The model under review builds one solid part; all positions refer to its coordinate system, in mm. A direction names the side the tool comes from. Round coordinates to 2 decimals unless told otherwise and drop trailing zeros. Write each loop counter-clockwise with the first axis right and the second up, starting at its lowest first coordinate (ties: lowest second). Pieces come first, ordered by that corner, then holes. Notation, with made-up numbers: M -25.5,31.5 L -5.5,31.5 A28 cw -5.5,56.5 Z; hole C -11.75,30 d10. An arc over 180 degrees is marked long. Write item = value, one per line. Start each with the question number.
Item 1: For pin 1 Ø4 at (x, z) = (-106, -24.5) entering from -Y (3 decimals); pin 2 Ø14.5 at (x, y) = (-106, -23) entering from -Z (3 decimals), all flat-tipped, find the tip position at first contact; note any pin that passes through.
Item 2: Take a section at A-A, the plane x = -50. Give the boundary of the cut face in (y, z) (3 decimals), plus the area to 3 significant figures.
Item 3: The part is to be moulded in two halves that separate along Z. For faces 1 (the cylindrical face through (-53.485, -11.949, -1.61)), 2 (the flat face through (3, -20, 0)), 3 (the flat face through (3, -21, -3.175)), 4 (the cylindrical face through (2.86, -1.61, -24.96)), say which applies: +Z half, -Z half, draft (parallel to the pull), parting line (faces both ways), or undercut.
Item 4: Take a section at B-B, the plane x = 109. Give the boundary of the cut face in (y, z) (3 decimals).
Item 5: To check wall thickness, follow line 1 along Y through (x, z) = (-182.5, -12) (3 decimals); line 2 along Y through (x, z) = (-204, -1). State the ranges of each line that lie inside material, in increasing order.
Item 6: Tool access review of faces 5 (the cylindrical face through (-52.172, -45.633, -1.61)), 6 (the flat face through (3, -3.175, -27)): name each direction out of +Z, -Z, +X, -X, +Y, -Y from which nothing blocks a thin tool from reaching the whole face with its end or side.
from build123d import *

# Parameters (mm, degrees)
BOSS_EXTRUDE1_DEPTH = 214.63
SKETCH2_R           = 2.5
SKETCH2_R_2         = 3.57
CUT_EXTRUDE1_DEPTH  = 223.403254304
CUT_EXTRUDE2_DEPTH  = 3.175
SKETCH4_R           = 2.5
CUT_EXTRUDE3_DEPTH  = 3.175
CUT_EXTRUDE4_REACH  = 224.131
SKETCH5_R           = 9.525
SKETCH6_R           = 2.6
CUT_EXTRUDE5_DEPTH  = 3.175


with BuildPart() as part:
    # Sketch1 → Boss-Extrude1 (new, symmetric)
    with BuildSketch(Plane(origin=(0, 0, 0), x_dir=(0, 0, -1), z_dir=(1, 0, 0))):
        Polygon((0, 0), (31.75, 0), (31.75, -3.175), (3.175, -3.175), (3.175, -50.8), (0, -50.8), align=None)
    extrude(amount=BOSS_EXTRUDE1_DEPTH, both=True)

    # Sketch2 → Cut-Extrude1 (cut, through all)
    with BuildSketch(Plane(origin=(0, 0, -3.175), x_dir=(-1, 0, 0), z_dir=(0, 0, -1))):
        with Locations(Location((-50, -11.175, 0), (0, 0, 90))):
            Circle(SKETCH2_R)
        with Locations(Location((50, -11.175, 0), (0, 0, 90))):
            Circle(SKETCH2_R_2)
        with Locations(Location((50, -42.8, 0), (0, 0, 90))):
            Circle(SKETCH2_R_2)
        with Locations(Location((-50, -42.8, 0), (0, 0, 90))):
            Circle(SKETCH2_R)
    extrude(amount=-CUT_EXTRUDE1_DEPTH, mode=Mode.SUBTRACT)

    # Sketch3 → Cut-Extrude2 (cut)
    with BuildSketch(Plane(origin=(0, 0, -3.175), x_dir=(-1, 0, 0), z_dir=(0, 0, -1))):
        Polygon((214.63, -50.8), (100.33, -50.8), (214.63, -23.175), align=None)
        Polygon((-214.63, -23.175), (-214.63, -50.8), (-100.33, -50.8), align=None)
    extrude(amount=-CUT_EXTRUDE2_DEPTH, mode=Mode.SUBTRACT)

    # Sketch4 → Cut-Extrude3 (cut)
    with BuildSketch(Plane(origin=(0, 0, 0), x_dir=(1, 0, 0), z_dir=(0, 1, 0))):
        with Locations(Location((-204.63, 11.176, 0), (0, 0, 270))):
            Circle(SKETCH4_R)
        with Locations(Location((-204.63, 25.176, 0), (0, 0, 270))):
            Circle(SKETCH4_R)
        with Locations(Location((204.63, 25.176, 0), (0, 0, 90))):
            Circle(SKETCH4_R)
        with Locations(Location((204.63, 11.176, 0), (0, 0, 90))):
            Circle(SKETCH4_R)
    extrude(amount=-CUT_EXTRUDE3_DEPTH, mode=Mode.SUBTRACT)

    # Sketch5 → Cut-Extrude4 (cut, up to next)
    with BuildSketch(Plane.XZ.offset(3.175), mode=Mode.PRIVATE) as cut_extrude4_sk1:
        with Locations(Location((0, -15.875, 0), (0, 0, 270))):
            Circle(SKETCH5_R)
    cut_extrude4_tool1 = extrude(cut_extrude4_sk1.sketch, amount=-CUT_EXTRUDE4_REACH, mode=Mode.PRIVATE) & part.part
    add(cut_extrude4_tool1.solids().sort_by_distance((0, -3.175, -15.875))[0], mode=Mode.SUBTRACT)

    # Sketch6 → Cut-Extrude5 (cut)
    with BuildSketch(Plane.XY):
        with Locations((204.63, -13.175000066)):
            Circle(SKETCH6_R)
        with Locations(Location((-204.63, -13.175000066, 0), (0, 0, 270))):
            Circle(SKETCH6_R)
    extrude(amount=-CUT_EXTRUDE5_DEPTH, mode=Mode.SUBTRACT)


solid = part.part
Response values:
q1.pin_1 = -3.175
q1.pin_2 = -3.175
q2.outline = M -50.8,-3.175 L -46.37,-3.175 L -46.37,0 L -50.8,0 Z; M -39.23,-3.175 L -14.745,-3.175 L -14.745,0 L -39.23,0 Z; M -7.605,-3.175 L -3.175,-3.175 L -3.175,-31.75 L 0,-31.75 L 0,0 L -7.605,0 Z
q2.area = 207 mm2
q3.face_1 = draft
q3.face_2 = +Z half
q3.face_3 = -Z half
q3.face_4 = undercut
q4.outline = M -48.705,-3.175 L -3.175,-3.175 L -3.175,-31.75 L 0,-31.75 L 0,0 L -48.705,0 Z
q5.line_1 = -3.175 to 0
q5.line_2 = -25.74 to -15.7, -10.65 to 0
q6.face_5 = +Z, -Z
q6.face_6 = -Z, +X, -X, -Y
